```python
from build123d import *

# Parameters (mm, degrees)
F1_DEPTH = 3
F3_DEPTH = 4


with BuildPart() as f1:
    # F0 (on Top) → F1 (new body)
    with BuildSketch(Plane.XY):
        with BuildLine():
            Line((32.444928, 31.685156), (74.762845, 73.012102))
            ThreePointArc((74.762845, 73.012102), (-39.417843, 96.780595), (-104.5, 0))
            Line((-104.5, 0), (-45.35, 0))
            ThreePointArc((-45.35, 0), (-17.106212, 42), (32.444928, 31.685156))
        make_face()
    extrude(amount=F1_DEPTH)

    # F2 (on face) → F3 (join)
    with BuildSketch(Plane.XY.offset(3)):
        Polygon((-24.734859, 59.074202), (-24.153877, 59.303767), (-24.908327, 61.156129), (-25.46983, 60.93426), align=None)
        Polygon((-24.908327, 61.156129), (-24.153877, 59.303767), (-22.874801, 59.809172), (-21.014742, 60.544143), (-21.749713, 62.404202), (-23.609771, 61.669231), align=None)
        Polygon((-30.247139, 73.024641), (-29.812251, 73.19648), (-30.566701, 75.048842), (-30.98211, 74.8847), align=None)
        Polygon((-30.566701, 75.048842), (-29.812251, 73.19648), (-28.387081, 73.759612), (-26.527022, 74.494583), (-27.261993, 76.354641), (-29.122051, 75.619671), align=None)
        Polygon((-55.841003, 34.054731), (-54.724372, 35.713989), (-56.383629, 36.83062), (-57.50026, 35.171363), align=None)
        Polygon((-68.285433, 42.429465), (-67.168802, 44.088722), (-68.828059, 45.205353), (-69.94469, 43.546096), align=None)
        Polygon((-68.828059, 45.205353), (-67.168802, 44.088722), (-66.052171, 45.747979), (-67.711428, 46.86461), align=None)
        Polygon((-56.383629, 36.83062), (-54.724372, 35.713989), (-53.60774, 37.373246), (-55.266998, 38.489877), align=None)
        Polygon((-56.957634, 32.395474), (-55.841003, 34.054731), (-57.50026, 35.171363), (-58.616891, 33.512105), align=None)
        Polygon((-69.402064, 40.770207), (-68.285433, 42.429465), (-69.94469, 43.546096), (-71.061321, 41.886838), align=None)
        Polygon((22.776784, 77.747336), (20.827569, 78.195176), (20.379729, 76.245961), (22.328944, 75.798121), align=None)
        Polygon((19.417982, 63.128223), (17.468767, 63.576063), (17.020927, 61.626848), (18.970142, 61.179008), align=None)
    extrude(amount=-F3_DEPTH)


solid = f1.part
```
Geometry check sheet. Reference: the model listing, model coordinates, mm. Give positions to 0.01 mm unless a question says otherwise; leave off trailing zeros. Write each loop counter-clockwise with the first axis right and the second up, starting at its lowest first coordinate (ties: lowest second). Pieces come first, ordered by that corner, then holes. Notation, with made-up numbers: (-13.75, 32.5) -> (22.25, 32.5) arc R19 ccw to (22.25, 38.5) -> close; hole circle Ø10 at (14.25, 77.5). An arc over 180 degrees is marked (long way). One line per question, with ' | ' between items.
Item 1: Scan lines: line 1 along Z through (x, y) = (-42, 44); line 2 along X through (y, z) = (35, 0.25); line 3 along Y through (x, z) = (50, 1). Record each from-to range of solid material in increasing order.
Determined:
line 1: 0 to 3 | line 2: -98.46 to -28.84, 28.84 to 35.84 | line 3: 48.83 to 91.76
Item 2: Sectioned sample at A-A, the plane z = 0.7. Record the boundary of the cut face in (x, y), plus the area to 3 significant figures.
Determined:
outline: (-104.5, 0) -> (-45.35, 0) arc R45.35 cw to (32.44, 31.69) -> (74.76, 73.01) arc R104.5 ccw to start | area: 10,500 mm^2
Item 3: Depth check by flat-ended pin: pin 1 (8 mm diameter, centred on x = 25, y = 69.5, fed in from -Z); pin 2 (1 mm diameter, centred on y = 40.5, z = 0.5, fed in from -X); pin 3 (2 mm diameter, centred on y = 51, z = 1.5, fed in from +X). Enter the tip coordinate at first touch or a pass-through.
Determined:
pin 1: z = 0 | pin 2: x = -96.54 | pin 3: x = 53.25
Item 4: Sectioned sample at B-B, the plane x = 0.5. Record the boundary of the cut face in (y, z).
Determined:
outline: (45.35, 0) -> (104.5, 0) -> (104.5, 3) -> (45.35, 3) -> close
